Build history of the part. All positions in model axes, mm. Give positions to 0.01 mm unless a question says otherwise; leave off trailing zeros. Order: outer loops, then holes, each group sorted by start corner. A loop starts at its lowest first (then second) coordinate and runs counter-clockwise, first axis right, second up. Notation, with made-up numbers: M 35,-26 L 73,-26 A7 ccw 73,-22 Z; hole C -14.5,-10.75 d2. An arc over 180 degrees is marked long. Answer as CSV lines item,"result".
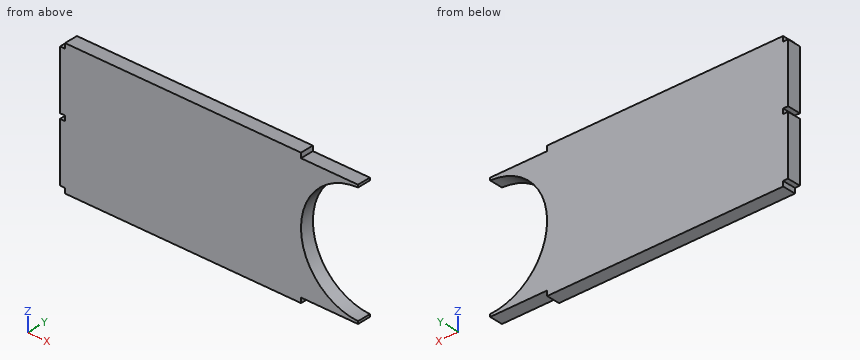
from build123d import *

# Parameters (mm, degrees)
SKETCH1_W           = 121.5
SKETCH1_H           = 54
BOSS_EXTRUDE1_DEPTH = 5.4864
SKETCH2_W           = 2
SKETCH2_H           = 2
SKETCH2_W_2         = 23.254
CUT_EXTRUDE1_DEPTH  = 67.705794988


with BuildPart() as part:
    # Sketch1 → Boss-Extrude1 (new body)
    with BuildSketch(Plane(origin=(0, 0, 0), x_dir=(1, 0, 0), z_dir=(0, 1, 0))):
        Rectangle(SKETCH1_W, SKETCH1_H)
    extrude(amount=BOSS_EXTRUDE1_DEPTH)

    # Sketch2 → Cut-Extrude1 (cut, through all)
    with BuildSketch(Plane(origin=(0, 5.4864, 0), x_dir=(1, 0, 0), z_dir=(0, 1, 0))):
        with Locations((-59.75, 0)):
            Rectangle(SKETCH2_W, SKETCH2_H)
        with Locations((-59.75, 26)):
            Rectangle(SKETCH2_W, SKETCH2_H)
        with Locations((-59.75, -26)):
            Rectangle(SKETCH2_W, SKETCH2_H)
        with Locations((49.123, 26)):
            Rectangle(SKETCH2_W_2, SKETCH2_H)
        with Locations((49.123, -26)):
            Rectangle(SKETCH2_W_2, SKETCH2_H)
        with BuildLine():
            Line((60.75, 23.988403115), (60.75, -23.988403115))
            ThreePointArc((60.75, -23.988403115), (37.496, 0), (60.75, 23.988403115))
        make_face()
    extrude(amount=-CUT_EXTRUDE1_DEPTH, mode=Mode.SUBTRACT)


solid = part.part
Item 1: Drop flat-ended pins along their axis: pin 1 (1.5 mm diameter, centred on y = 1, z = 11, fed in from +X); pin 2 (1 mm diameter, centred on y = 1.5, z = 26, fed in from -X); pin 3 (2 mm diameter, centred on x = -60, y = 4, fed in from +Z). Give the stop position or say it passes through.
Geometry says:
pin 1,"stops at x = 40.57"
pin 2,"stops at x = -58.75"
pin 3,"stops at z = 25"
Item 2: Band-saw the part on A-A (y = 1.65). Give the cut face in (x, z).
Geometry says:
outline,"M -60.75,-25 L -58.75,-25 L -58.75,-27 L 37.5,-27 L 37.5,-25 L 60.75,-25 L 60.75,-23.99 A24 cw 60.75,23.99 L 60.75,25 L 37.5,25 L 37.5,27 L -58.75,27 L -58.75,25 L -60.75,25 L -60.75,1 L -58.75,1 L -58.75,-1 L -60.75,-1 Z"
Item 3: Band-saw the part on C-C (z = 4.5). Give the cut face in (x, y).
Geometry says:
outline,"M -60.75,0 L 37.92,0 L 37.92,5.49 L -60.75,5.49 Z"
Item 4: Band-saw the part on B-B (z = -7). Give the cut face in (x, y), and give its area (3 significant figures).
Geometry says:
outline,"M -60.75,0 L 38.54,0 L 38.54,5.49 L -60.75,5.49 Z"
area,"545 mm2"
Item 5: Probe line 1 along Z through (x, y) = (44.5, 2.8); line 2 along Z through (x, y) = (55.5, 3.95); line 3 along X through (y, z) = (1.3, -18.5). List the from-to ranges inside material, lowest first. Write a range as from..to.
Geometry says:
line 1,"z = -25..-16.95, 16.95..25"
line 2,"z = -25..-23.24, 23.24..25"
line 3,"x = -60.75..46.21"
